from build123d import *

# Parameters (mm, degrees)
MODEL_R             = 14.2875
MODEL_R_2           = 3.175
BOSS_EXTRUDE1_DEPTH = 6.35
SKETCH2_W           = 177.682226564
SKETCH2_H           = 158.75
CUT_EXTRUDE1_DEPTH  = 6.35


with BuildPart() as part:
    # Model → Boss-Extrude1 (new body)
    with BuildSketch(Plane.XY):
        with BuildLine():
            Line((0, 304.8), (-406.4, 304.8))
            Line((-406.4, 304.8), (-406.4, -120.65))
            Line((-406.4, -120.65), (-406.4, -138.610512242))
            Line((-406.4, -138.610512242), (-240.210512242, -304.8))
            Line((-240.210512242, -304.8), (-222.25, -304.8))
            Line((-222.25, -304.8), (0, -304.8))
            ThreePointArc((0, -304.8), (304.8, 0), (0, 304.8))
        make_face()
        with Locations((-282.557162358, 114.3)):
            Circle(MODEL_R, mode=Mode.SUBTRACT)
        with Locations((-179.408571771, 114.3)):
            Circle(MODEL_R, mode=Mode.SUBTRACT)
        with Locations((0, 114.3)):
            Circle(MODEL_R, mode=Mode.SUBTRACT)
        with Locations((80.82230509, 80.82230509)):
            Circle(MODEL_R, mode=Mode.SUBTRACT)
        with Locations((114.3, 0)):
            Circle(MODEL_R, mode=Mode.SUBTRACT)
        with Locations((80.82230509, -80.82230509)):
            Circle(MODEL_R, mode=Mode.SUBTRACT)
        with Locations((0, -114.3)):
            Circle(MODEL_R, mode=Mode.SUBTRACT)
        with Locations((-179.316283411, -118.368022334)):
            Circle(MODEL_R, mode=Mode.SUBTRACT)
        with Locations((-381, -120.65)):
            Circle(MODEL_R, mode=Mode.SUBTRACT)
        with Locations((-279.904657875, -120.65)):
            Circle(MODEL_R, mode=Mode.SUBTRACT)
        Circle(MODEL_R, mode=Mode.SUBTRACT)
        with Locations((57.15, 0)):
            Circle(MODEL_R, mode=Mode.SUBTRACT)
        with Locations((37.893602924, 107.835823628)):
            Circle(MODEL_R_2, mode=Mode.SUBTRACT)
        with Locations((107.090214294, 39.952171435)):
            Circle(MODEL_R_2, mode=Mode.SUBTRACT)
        with Locations((107.090214294, -39.952171435)):
            Circle(MODEL_R_2, mode=Mode.SUBTRACT)
        with Locations((-327.981609649, 112.531845238)):
            Circle(MODEL_R_2, mode=Mode.SUBTRACT)
        with Locations((-330.785746456, -114.289302148)):
            Circle(MODEL_R_2, mode=Mode.SUBTRACT)
        with Locations((-228.6, 114.3)):
            Circle(MODEL_R_2, mode=Mode.SUBTRACT)
        with Locations((-127, 114.3)):
            Circle(MODEL_R_2, mode=Mode.SUBTRACT)
        with Locations((-76.2, 114.3)):
            Circle(MODEL_R_2, mode=Mode.SUBTRACT)
        with Locations((-76.2, -114.3)):
            Circle(MODEL_R_2, mode=Mode.SUBTRACT)
        with Locations((-127, -114.3)):
            Circle(MODEL_R_2, mode=Mode.SUBTRACT)
        with Locations((-228.6, -114.3)):
            Circle(MODEL_R_2, mode=Mode.SUBTRACT)
    extrude(amount=BOSS_EXTRUDE1_DEPTH)

    # Sketch2 → Cut-Extrude1 (cut)
    with BuildSketch(Plane.XY.offset(6.35)):
        with Locations((-317.558886718, 225.425)):
            Rectangle(SKETCH2_W, SKETCH2_H)
    extrude(amount=-CUT_EXTRUDE1_DEPTH, mode=Mode.SUBTRACT)


solid = part.part
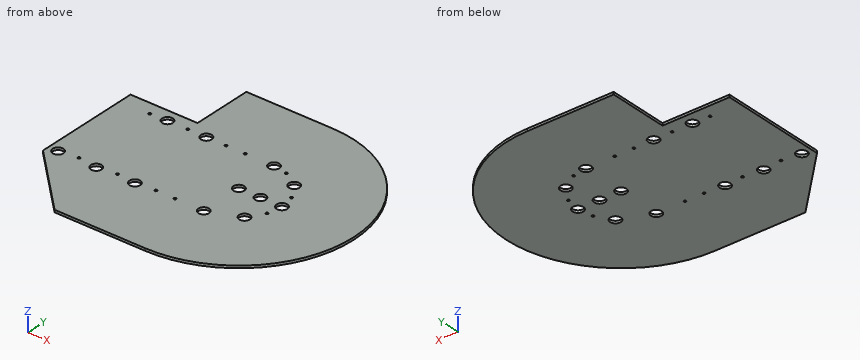
Verification items for the finished model (mm, model axes). Coordinates: 2 decimals unless noted, no trailing zeros. Order: outer loops, then holes, each group sorted by start corner. A loop starts at its lowest first (then second) coordinate and runs counter-clockwise, first axis right, second up. Notation, with made-up numbers: M 29,-15 L 73,-15 A25 cw 73,9 Z; hole C -22,-19 d2. An arc over 180 degrees is marked long. One line per item, written item: value. Start each with the question number.
Item 1: Thickness scan on probe 1 along Y at (x, z) = (-127, 4.75) (3 decimals); probe 2 along Y at (x, z) = (0, 1.5); probe 3 along Y at (x, z) = (-278.5, 1.5). Record the ranges inside material, lowest first.
Item 2: Sectioned sample at C-C on x = 57.15. Record the cut outline in (y, z), then the cut area to 3 significant figures.
Item 3: Depth check by flat-ended pin: P1, Ø3, axis at x = -285, z = 2.5, coming from the +Y side; P2, Ø3, axis at y = -207, z = 0.5, coming from the -X side; P3, Ø1.9, axis at y = 225.5, z = 2, coming from the -X side. Enter the tip coordinate at first touch or a pass-through.
Item 4: Sectioned sample at D-D on y = 234.5. Record the cut outline in (x, z).
Item 5: Sectioned sample at A-A on y = 0. Record the cut outline in (x, z), then the cut area to 3 significant figures.
Item 6: Sectioned sample at B-B on z = 2. Give the number of separate pieces and of enclosed holes in the cut face, then the cut area to 3 significant figures.
Calculated:
1. probe 1: -304.8 to -117.475, -111.125 to 111.125, 117.475 to 304.8
1. probe 2: -304.8 to -128.59, -100.01 to -14.29, 14.29 to 100.01, 128.59 to 304.8
1. probe 3: -266.51 to -134.87, -106.43 to 100.6, 128 to 146.05
2. outline: M -299.39,0 L -14.29,0 L -14.29,6.35 L -299.39,6.35 Z; M 14.29,0 L 299.39,0 L 299.39,6.35 L 14.29,6.35 Z
2. area: 3,620 mm^2
3. P1: y = 146.05
3. P2: x = -339.51
3. P3: x = -228.72
4. outline: M -228.72,0 L 194.71,0 L 194.71,6.35 L -228.72,6.35 Z
5. outline: M -406.4,0 L -14.29,0 L -14.29,6.35 L -406.4,6.35 Z; M 14.29,0 L 42.86,0 L 42.86,6.35 L 14.29,6.35 Z; M 71.44,0 L 100.01,0 L 100.01,6.35 L 71.44,6.35 Z; M 128.59,0 L 304.8,0 L 304.8,6.35 L 128.59,6.35 Z
5. area: 3,970 mm^2
6. separate pieces: 1
6. enclosed holes: 23
6. area: 344,000 mm^2
